from build123d import *

# Parameters (mm, degrees)
F0_R     = 2.75
F0_R_2   = 1.5
F1_DEPTH = 9
F0_R_3   = 3.4
F2_DEPTH = 1
F0_R_4   = 4.8
F3_DEPTH = 20
F4_SIZE  = 1
F5_SIZE  = 0.3


with BuildPart() as f1:
    # F0 (on Top) → F1 (new body)
    with BuildSketch(Plane.XY):
        Circle(F0_R)
        Circle(F0_R_2, mode=Mode.SUBTRACT)
    extrude(amount=-F1_DEPTH)

    # F0 (on Top) → F2 (join)
    with BuildSketch(Plane.XY):
        Circle(F0_R_3)
        Circle(F0_R, mode=Mode.SUBTRACT)
        Circle(F0_R)
        Circle(F0_R_2, mode=Mode.SUBTRACT)
    extrude(amount=F2_DEPTH)

    # F0 (on Top) → F3 (join)
    with BuildSketch(Plane.XY):
        Circle(F0_R_4)
        Circle(F0_R_3, mode=Mode.SUBTRACT)
    extrude(amount=F3_DEPTH)

    # F4
    f4_edges = [f1.edges().sort_by_distance(p)[0] for p in [
        (-4.8, 0, 0),
    ]]
    chamfer(f4_edges, length=F4_SIZE)

    # F5
    f5_edges = [f1.edges().sort_by_distance(p)[0] for p in [
        (-1.5, 0, 1),
    ]]
    chamfer(f5_edges, length=F5_SIZE)


solid = f1.part
The listing builds one solid part. Answer for the finished solid, in the listing's coordinates (mm). A direction names the side the tool comes from. Coordinates: 2 decimals unless noted, no trailing zeros. Loops run counter-clockwise (first coordinate to the right, second up) from the corner with the lowest first, then second, coordinate; pieces in that order, holes last.
1) Determine the mould class of faces 1 (the face through (-1.5, 0.07, -4.22)), 2 (the face through (3, 1, 0)), 3 (the face through (-0.74, -3.32, 10.37)), 4 (the face through (-0.596, -2.685, -4.437)) for opening direction X: pulls with the +X half, pulls with the -X half, needs draft (parallel to the pull), parting line crosses it, or undercut.
2) Find the intervals of material crossed by L1, parallel to Y at x = 0, z = 7.25; L2, parallel to Y at x = 0, z = -5.75; L3, parallel to X at y = 0.5, z = 11, in increasing order.
3) Find section C-C on z = 17. Write down the section's boundary in (x, y), then the cut area to 3 significant figures.
4) A tool of negligible diameter and unlimited length cuts with its end or side. For faces 5 (the face through (2.58, 4.05, 10.37)), 6 (the face through (1.5, -1.5, 1)), from which of +Z, -Z, +X, -X, +Y, -Y can it reach the whole face along a straight path? Write none if from no direction.
5) Flat-ended cylindrical pins translate along their axes: pin 1 Ø1.8 at (x, y) = (0, 0) entering from +Z; pin 2 Ø4 at (x, z) = (2.5, 10) entering from -Y. Find the tip coordinate at first contact, or state that the pin passes through.
6) Find section D-D on z = -6.25. Write down the section's boundary in (x, y).
7) Find section A-A on y = 0. Write down the section's boundary in (x, z), then the cut area to 3 significant figures.
Values:
1. face 1: undercut
1. face 2: needs draft
1. face 3: undercut
1. face 4: parting line crosses it
2. L1: y = -4.8 to -3.4, 3.4 to 4.8
2. L2: y = -2.75 to -1.5, 1.5 to 2.75
2. L3: x = -4.77 to -3.36, 3.36 to 4.77
3. outline: circle Ø9.6 at (0, 0); hole circle Ø6.8 at (0, 0)
3. area: 36.1 mm2
4. face 5: +Z, -Z
4. face 6: +Z
5. pin 1: passes through
5. pin 2: stops at y = -4.77
6. outline: circle Ø5.5 at (0, 0); hole circle Ø3 at (0, 0)
7. outline: (-4.8, 1) - (-3.8, 0) - (-2.75, 0) - (-2.75, -9) - (-1.5, -9) - (-1.5, 0.7) - (-1.8, 1) - (-3.4, 1) - (-3.4, 20) - (-4.8, 20) - close; (1.5, -9) - (2.75, -9) - (2.75, 0) - (3.8, 0) - (4.8, 1) - (4.8, 20) - (3.4, 20) - (3.4, 1) - (1.8, 1) - (1.5, 0.7) - close
7. area: 81.2 mm2
